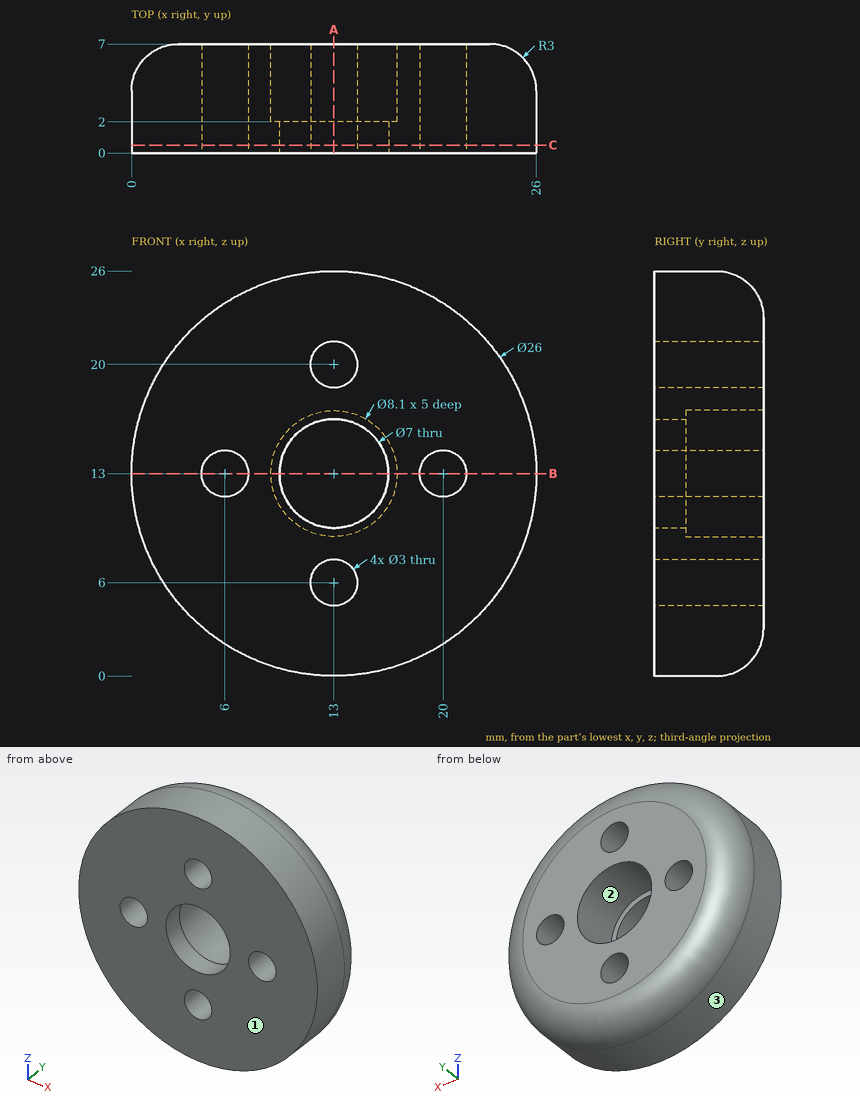
Verification items for this drawing (mm, ordinates from the low corner). Round coordinates to 2 decimals unless told otherwise and drop trailing zeros. Order: outer loops, then holes, each group sorted by start corner. A loop starts at its lowest first (then second) coordinate and runs counter-clockwise, first axis right, second up. Notation, with made-up numbers: (-1, 87) -> (37, 87) arc R18 ccw to (37, 100) -> close; hole circle Ø2 at (49, 85.5). An arc over 180 degrees is marked (long way). Use one line per item in the form item = value.
1. Go/stop test with flat-tipped pins: pin 1 (11 mm diameter, centred on x = 13, z = 13, fed in from +Y); pin 2 (3 mm diameter, centred on x = 15, y = 5.5, fed in from +Z); pin 3 (1.5 mm diameter, centred on y = 1.5, z = 19.5, fed in from +X); pin 4 (4 mm diameter, centred on x = 3.5, y = 6.5, fed in from -Z). Record where each tip stops, or that it passes through.
Working result:
pin_1 = 7
pin_2 = 25.94
pin_3 = 24.66
pin_4 = 3.05
2. Cross-section at C-C, the plane y = 0.5. Enter the section's corners in (x, z).
Working result:
outline = circle Ø26 at (13, 13); hole circle Ø3 at (6, 13); hole circle Ø7 at (13, 13); hole circle Ø3 at (13, 6); hole circle Ø3 at (13, 20); hole circle Ø3 at (20, 13)
3. Cross-section at A-A, the plane x = 13. Enter the section's corners in (y, z), plus the area to 3 significant figures.
Working result:
outline = (0, 0) -> (4, 0) arc R3 ccw to (7, 3) -> (7, 4.5) -> (0, 4.5) -> close; (0, 7.5) -> (7, 7.5) -> (7, 8.95) -> (2, 8.95) -> (2, 9.5) -> (0, 9.5) -> close; (0, 16.5) -> (2, 16.5) -> (2, 17.05) -> (7, 17.05) -> (7, 18.5) -> (0, 18.5) -> close; (0, 21.5) -> (7, 21.5) -> (7, 23) arc R3 ccw to (4, 26) -> (0, 26) -> close
area = 81.6 mm^2
4. Scan lines: line 1 along X through (y, z) = (2.25, 13); line 2 along X through (y, z) = (1.75, 13); line 3 along Z through (x, y) = (13.5, 6). Record each from-to range of solid material in increasing order. Write a range as from..to.
Working result:
line_1 = 0..4.5, 7.5..8.95, 17.05..18.5, 21.5..26
line_2 = 0..4.5, 7.5..9.5, 16.5..18.5, 21.5..26
line_3 = 0.77..4.59, 7.41..8.98, 17.02..18.59, 21.41..25.23
5. Cross-section at B-B, the plane z = 13. Enter the section's corners in (x, y), plus the area to 3 significant figures.
Working result:
outline = (0, 0) -> (4.5, 0) -> (4.5, 7) -> (3, 7) arc R3 ccw to (0, 4) -> close; (7.5, 0) -> (9.5, 0) -> (9.5, 2) -> (8.95, 2) -> (8.95, 7) -> (7.5, 7) -> close; (16.5, 0) -> (18.5, 0) -> (18.5, 7) -> (17.05, 7) -> (17.05, 2) -> (16.5, 2) -> close; (21.5, 0) -> (26, 0) -> (26, 4) arc R3 ccw to (23, 7) -> (21.5, 7) -> close
area = 81.6 mm^2
6. Mould release check, pull along Z, two halves, no side actions. Record for the marked faces 1, 2 and 3: pulls with the +Z half, pulls with the -Z half, needs draft (parallel to the pull), parting line crosses it, or undercut.
Working result:
face_1 = needs draft
face_2 = undercut
face_3 = parting line crosses it
